Check sheet for the modelled part. Datum: model origin and axes. Units: mm. A direction names the side the tool comes from. Give positions to 0.01 mm unless a question says otherwise; leave off trailing zeros. Loops run counter-clockwise (first coordinate to the right, second up) from the corner with the lowest first, then second, coordinate; pieces in that order, holes last. Notation, with made-up numbers: M 26.5,57 L 55.5,57 A36 cw 55.5,92 Z; hole C 45.25,-37.5 d3. An arc over 180 degrees is marked long. One line per question, with ' | ' between items. Start each with the question number.
from build123d import *

# Parameters (mm, degrees)
BOSS_EXTRUDE1_DEPTH  = 30
FILLET3_R            = 5
M8_CLEARANCE_HOLE2_D = 9


with BuildPart() as part:
    # Sketch1 → Boss-Extrude1 (new body)
    with BuildSketch(Plane.XY):
        with BuildLine():
            Line((0, 5), (0, 0))
            Line((0, 0), (50, 0))
            ThreePointArc((50, 0), (54.964763693, 2.630857457), (55.575665525, 8.216292841))
            ThreePointArc((55.575665525, 8.216292841), (71.373384511, 31.495789225), (87.171103497, 8.216292841))
            ThreePointArc((87.171103497, 8.216292841), (87.782005329, 2.630857457), (92.746769021, 0))
            Line((92.746769021, 0), (142.746769021, 0))
            Line((142.746769021, 0), (142.746769021, 5))
            Line((142.746769021, 5), (91.218534724, 5))
            ThreePointArc((91.218534724, 5), (71.373384511, 36.495789225), (51.528234297, 5))
            Line((51.528234297, 5), (5, 5))
            Line((5, 5), (0, 5))
        make_face()
    extrude(amount=BOSS_EXTRUDE1_DEPTH)

    # Fillet3
    fillet3_edges = [part.edges().sort_by_distance(p)[0] for p in [
        (51.528234297, 5, 15),
        (91.218534724, 5, 15),
    ]]
    fillet(fillet3_edges, radius=FILLET3_R)

    # M8 Clearance Hole2 (through all)
    with Locations(Plane(origin=(0, 5, 0), x_dir=(1, 0, 0), z_dir=(0, 1, 0))):
        with Locations((20, -15), (122.746769021, -15)):
            Hole(M8_CLEARANCE_HOLE2_D / 2)


solid = part.part
Q1. Cross-section at B-B (x = 20). Record the cut outline in (y, z).
Q2. Material ranges on probe 1 along Z at (x, y) = (20, 3.25); probe 2 along Y at (x, z) = (132.5, 23.75); probe 3 along X at (y, z) = (20, 9.25), recorded low to high. Write a range as from..to.
Q3. Draft check along Y on faces 4 (the flat face through (28, 5, 15)), 5 (the flat face through (0, 3, 15)), 6 (the cylindrical face through (54.918, 2.563, 14.79)), 7 (the cylindrical face through (94.217, 6.726, 15.21)). Enter one of: released by +Y, released by -Y, zero draft, split by the parting line, or undercut.
Q4. Cross-section at A-A (y = 3). Record the cut outline in (x, z).
Q5. Cross-section at C-C (z = 18.25). Record the cut outline in (x, y).
Q6. Cross-section at D-D (y = 18). Record the cut outline in (x, z), and give its area (3 significant figures).
Q7. Depth check by flat-ended pin: P1, Ø1, axis at x = 64.5, z = 7, coming from the -Y side; P2, Ø12, axis at y = 24.5, z = 14.5, coming from the +X side; P3, Ø15, axis at x = 130.5, z = 16, coming from the +Y side. Enter the tip coordinate at first touch or a pass-through.
Q8. Access from +Z, -Z, +X, -X, +Y, -Y to the whole of each face (thin tool, end or side, straight path). Record for faces 1 (the flat face through (25, 0, 15)), 2 (the cylindrical face through (87.737, 2.699, 14.79)), 3 (the flat face through (116, 5, 15)).
Solved:
1) outline: M 0,0 L 5,0 L 5,10.5 L 0,10.5 Z; M 0,19.5 L 5,19.5 L 5,30 L 0,30 Z
2) probe 1: z = 0..10.5, 19.5..30 | probe 2: y = 0..5 | probe 3: x = 50.07..55.29, 87.46..92.67
3) face 4: released by +Y | face 5: zero draft | face 6: undercut | face 7: undercut
4) outline: M 0,0 L 55.2,0 L 55.2,30 L 0,30 Z; M 87.55,0 L 142.75,0 L 142.75,30 L 87.55,30 Z; hole C 20,15 d9; hole C 122.75,15 d9
5) outline: M 0,0 L 16.89,0 L 16.89,5 L 0,5 Z; M 23.11,0 L 50,0 A6 ccw 55.58,8.22 A17 cw long 87.17,8.22 A6 ccw 92.75,0 L 119.63,0 L 119.63,5 L 98,5 A5 cw 93.07,10.83 A22 ccw long 49.68,10.83 A5 cw 44.75,5 L 23.11,5 Z; M 125.86,0 L 142.75,0 L 142.75,5 L 125.86,5 Z
6) outline: M 49.65,0 L 54.74,0 L 54.74,30 L 49.65,30 Z; M 88.01,0 L 93.09,0 L 93.09,30 L 88.01,30 Z | area: 305 mm²
7) P1: stops at y = 29.81 | P2: stops at x = 93.01 | P3: stops at y = 5
8) face 1: +Z, -Z, +X, -X, -Y | face 2: +Z, -Z | face 3: +Z, -Z, +X, +Y
